Autodesk Inventor part; units mm, degrees
ref_plane "YZ Plane" through (0, 0, 0) normal (1, 0, 0) x (0, 1, 0)
ref_plane "XZ Plane" through (0, 0, 0) normal (0, 1, 0) x (-1, 0, 0)
ref_plane "XY Plane" through (0, 0, 0) normal (0, 0, 1) x (1, 0, 0)
sketch "スケッチ1" plane through (0, 0, 0) normal (0, 1, 0) x (-1, 0, 0)
  circle A0 centre (0, 0) radius 125
  dimension "d0" = 250
extrude "押し出し1" add sketch "スケッチ1" along normal blind 375
sketch "スケッチ2" plane through (0, 0, 0) normal (0, -1, 0) x (1, 0, 0)
  circle A0 centre (0, 0) radius 125
extrude "押し出し2" cut sketch "スケッチ2" against normal blind 40
sketch "スケッチ3" plane through (0, 40, 0) normal (0, -1, 0) x (1, 0, 0)
  circle A0 centre (0, 0) radius 125
  point P0 (0, 100)
  point P1 (-86.6025, -50)
  point P2 (86.6025, -50)
  dimension "d5" = 100
  dimension "d8" = 360
hole "穴1" at (0, 40, 100) at (-86.6025, 40, -50) at (86.6025, 40, -50) direction (0, 1, 0) diameter 3.2 depth 8
sketch "スケッチ4" plane through (0, 40, 0) normal (0, -1, 0) x (1, 0, 0)
  circle A0 centre (0, 100) radius 1.6
  point P0 (0, 0)
  point P1 (0, 110)
  point P2 (-95.2628, -55)
  point P3 (95.2628, -55)
  dimension "d17" = 10
  dimension "d20" = 360
hole "穴2" at (0, 40, 110) at (-95.2628, 40, -55) at (95.2628, 40, -55) direction (0, 1, 0) diameter 3.2 depth 8
sketch "スケッチ5" plane through (0, 375, 0) normal (0, 1, 0) x (1, 0, 0)
  circle A0 centre (0, 0) radius 120
  dimension "d29" = 240
extrude "押し出し3" cut sketch "スケッチ5" against normal blind 330
sketch "スケッチ6" plane through (0, 45, 0) normal (0, 1, 0) x (1, 0, 0)
  circle A0 centre (0, 0) radius 120
  line L0 (0, -118) -> (-21.8174, -118)
  line L1 (0, -118) -> (21.8174, -118)
  arc A1 (21.8174, -118) -> (-21.8174, -118) centre (0, 0) ccw
  arc A2 (-21.8174, -118) -> (21.8174, -118) centre (0, 0) ccw
  arc A3 (113.0997, 40.1056) -> (91.2823, 77.8944) centre (0, 0) ccw
  line L2 (102.191, 59) -> (91.2823, 77.8944)
  line L3 (102.191, 59) -> (113.0997, 40.1056)
  arc A4 (-91.2823, 77.8944) -> (-113.0997, 40.1056) centre (0, 0) ccw
  line L4 (-102.191, 59) -> (-113.0997, 40.1056)
  line L5 (-102.191, 59) -> (-91.2823, 77.8944)
  point P0 (-91.2823, 77.8944)
  point P1 (-113.0997, 40.1056)
  point P2 (113.0997, 40.1056)
  point P3 (91.2823, 77.8944)
  dimension "d32" = 118
  dimension "d35" = 360
extrude "押し出し4" add sketch "スケッチ6" along normal blind 330 contours L3 L2 A0 | A0 L0 L1 | L5 L4 A0
sketch "スケッチ8" plane through (21.8174, 45, 118) normal (0, 0, -1) x (-1, 0, 0)
  line L0 (43.6348, 0) -> (0, 0)
  point P0 (21.8174, -45)
  point P1 (11.8174, 60)
  point P2 (31.8174, 60)
  point P3 (11.8174, 90)
  point P4 (31.8174, 90)
  dimension "d52" = 30
  dimension "d90" = 60
  dimension "d91" = 60
  dimension "d92" = 30
hole "穴4" at (10, 105, 118) at (-10, 105, 118) at (10, 135, 118) at (-10, 135, 118) direction (0, 0, 1) diameter 3.2 depth 8
sketch "スケッチ11" plane through (113.0997, 45, -40.1056) normal (-0.8660254, 0, 0.5) x (0.5, 0, 0.8660254)
  line L0 (0, 0) -> (-43.6348, 0)
  point P0 (-21.8174, -45)
  point P1 (-31.8174, 60)
  point P2 (-31.8174, 90)
  point P3 (-11.8174, 60)
  point P4 (-11.8174, 90)
  dimension "d65" = 30
  dimension "d95" = 60
  dimension "d96" = 60
  dimension "d98" = 30
hole "穴5" at (97.191, 105, -67.6603) at (97.191, 135, -67.6603) at (107.191, 135, -50.3397) at (107.191, 105, -50.3397) direction (0.8660254, 0, -0.5) diameter 3.2 depth 8
sketch "スケッチ12" plane through (0, 375, 0) normal (0, 1, 0) x (1, 0, 0)
  circle A0 centre (0, 0) radius 121.5
  dimension "d73" = 243
extrude "押し出し6" cut sketch "スケッチ12" against normal blind 330
sketch "スケッチ13" plane through (0, 375, 0) normal (0, 1, 0) x (1, 0, 0)
  circle A0 centre (0, 0) radius 125
  line L0 (0, -125) -> (0, 0)
  line L1 (0, 0) -> (108.2532, 62.5)
  arc A1 (0, -125) -> (108.2532, 62.5) centre (0, 0) ccw
  circle A2 centre (0, 0) radius 125
  dimension "d76" = 125
  dimension "d77" = 120
extrude "押し出し7" cut sketch "スケッチ13" against normal blind 400 contours L1 L0 A0 picked at (69.3351, 45.9431)
sketch "スケッチ14" plane through (0, 45, 0) normal (0, 1, 0) x (1, 0, 0)
  line L0 (0, 0) -> (85.2169, 49.2)
  line L1 (0, -111.6) -> (0, -121.5)
  circle A0 centre (0, 0) radius 121.5
extrude "押し出し8" cut sketch "スケッチ14" against normal blind 400
sketch "スケッチ15" plane through (0, 40, 0) normal (0, -1, 0) x (1, 0, 0)
  line L0 (0, 0) -> (105.2221, 60.75)
  arc A0 (105.2221, -60.75) -> (0, 121.5) centre (0, 0) ccw
  line L1 (0, 0) -> (121.5, 0) construction
  line L2 (102.9357, 59.43) -> (115.531, 37.6143)
  line L3 (102.9357, 59.43) -> (90.3404, 81.2456)
  dimension "d82" = 30
extrude "押し出し9" add sketch "スケッチ15" against normal blind 335
sketch "スケッチ17" plane through (0, 40, 0) normal (0, -1, 0) x (1, 0, 0)
  circle A0 centre (0, 0) radius 125
extrude "押し出し11" cut sketch "スケッチ17" against normal blind 5
sketch "スケッチ19" plane through (0, 375, 0) normal (0, 1, 0) x (1, 0, 0)
  arc A0 (115.531, -37.6143) -> (105.2221, 60.75) centre (0, 0) ccw
  line L0 (115.531, -37.6143) -> (90.3404, -81.2456)
  line L1 (115.531, -37.6143) -> (90.3404, -81.2456)
  line L2 (90.3404, -81.2456) -> (81.6802, -76.2456)
  line L3 (115.531, -37.6143) -> (106.8708, -32.6143)
  line L4 (106.8708, -32.6143) -> (81.6802, -76.2456)
  dimension "d104" = 10
extrude "押し出し13" add sketch "スケッチ19" against normal blind 330
sketch "スケッチ21" plane through (0, 375, 0) normal (0, 1, 0) x (1, 0, 0)
  circle A0 centre (0, 0) radius 125
extrude "押し出し15" cut sketch "スケッチ21" against normal blind 230
fillet "フィレット1" radius 8 2 edges at (115.531, 95, 37.6143) (90.3404, 95, 81.2456)
sketch "スケッチ22" plane through (106.8708, 45, 32.6143) normal (-0.8660254, 0, -0.5) x (-0.5, 0, 0.8660254)
  line L0 (50.3812, 100) -> (0, 100)
  line L1 (25.1906, 85) -> (25.1906, 80.9836)
  point P0 (25.1906, -45)
  point P1 (10.1906, 85)
  point P2 (10.1906, 70)
  point P3 (40.1906, 85)
  point P4 (40.1906, 70)
  dimension "d112" = 15
  dimension "d113" = 15
  dimension "d114" = 15
hole "穴6" at (94.2755, 130, 54.43) at (101.7755, 130, 41.4396) at (101.7755, 115, 41.4396) at (86.7755, 130, 67.4204) at (86.7755, 115, 67.4204) direction (0.8660254, 0, 0.5) diameter 2.6 depth 10
sketch "スケッチ23" plane through (0, 45, 0) normal (0, -1, 0) x (1, 0, 0)
  line L0 (81.6802, 76.2456) -> (106.8708, 32.6143)
  arc A0 (118.386, 27.3315) -> (106.8708, 32.6143) centre (110.591, 25.5319) ccw
  line L1 (106.8708, 32.6143) -> (94.2755, 54.4299)
  line L2 (102.2857, 60.5558) -> (93.6255, 55.5558)
  line L3 (94.2755, 54.43) -> (101.2037, 58.43)
  line L4 (103.5857, 58.3041) -> (94.9255, 53.3041)
  line L5 (94.2755, 54.43) -> (102.2755, 54.43) construction
  point P0 (0, 0)
  dimension "d124" = 25.1905
  dimension "d126" = 8
  dimension "d127" = 30
hole "穴7" at (101.2037, 45, 58.43) direction (0, 1, 0) diameter 2.6 depth 10
sketch "スケッチ24" plane through (0, 45, 0) normal (0, -1, 0) x (1, 0, 0)
  circle A0 centre (101.2037, 58.43) radius 1.3
  line L0 (101.2037, 58.43) -> (96.2037, 67.0902)
  line L1 (94.7857, 73.5462) -> (86.1255, 68.5462)
  line L2 (101.2037, 58.43) -> (111.2037, 58.43) construction
  line L3 (96.2037, 67.0902) -> (106.2037, 49.7697)
  point P0 (0, 0)
  dimension "d135" = 10
  dimension "d136" = 120
  dimension "d137" = 20
hole "穴8" at (96.2037, 45, 67.0902) at (106.2037, 45, 49.7697) direction (0, 1, 0) diameter 2.6 depth 10
sketch "スケッチ27" plane through (0, 145, 0) normal (0, 1, 0) x (1, 0, 0)
  circle A0 centre (101.2037, -58.43) radius 1.3
  circle A1 centre (96.2037, -67.0902) radius 1.3
  circle A2 centre (106.2037, -49.7697) radius 1.3
  point P0 (0, 0)
hole "穴10" at (101.2037, 145, 58.43) at (96.2037, 145, 67.0902) at (106.2037, 145, 49.7697) direction (0, -1, 0) diameter 2.7 depth 10
properties part number "newbody5" material "PC/ABS プラスチック"
Geometry check sheet. Reference: the model listing, model coordinates, mm. A direction names the side the tool comes from. Give positions to 0.01 mm unless a question says otherwise; leave off trailing zeros. Loops run counter-clockwise (first coordinate to the right, second up) from the corner with the lowest first, then second, coordinate; pieces in that order, holes last. Notation, with made-up numbers: (66, 89) -> (99, 89) arc R25 ccw to (99, 124) -> close; hole circle Ø5 at (-15, 8). An arc over 180 degrees is marked (long way). Answer in a Markdown table with one row per item. Add a question column.
1) Cross-section at C-C on x = 48. Record the boundary of the cut face in (y, z), and give its area (3 significant figures).
2) Gauge pin test, flat ends, axial feed: P1, Ø2, axis at x = 101, z = 58.5, coming from the +Y side; P2, Ø1.5, axis at x = 82.5, y = 58, coming from the -Z side; P3, Ø12, axis at y = 70, z = 41, coming from the +X side. Record the tip position at first contact, or that the pin passes through.
3) Cross-section at A-A on y = 63. Record the boundary of the cut face in (x, z).
4) Material ranges on probe 1 along Y at (x, z) = (94, 72); probe 2 along Y at (x, z) = (10, 122); probe 3 along X at (y, z) = (98, -2.5) (3 decimals), recorded low to high. Write a range as from..to.
5) Draft check along Y on faces 1 (the face through (99, 45, 52)), 2 (the face through (85.357, 94.3, 82.166)), 3 (the face through (110.723, 104.14, -53.937)), 4 (the face through (99, 145, 52)). Enter one of: pulls with the +Y half, pulls with the -Y half, needs draft (parallel to the pull), parting line crosses it, or undercut.
6) Set-up check for faces 5 (the face through (98.47, 131.24, 57.3)), 6 (the face through (114.022, 94.3, 32.753)): record each of +Z, -Z, +X, -X, +Y, -Y from which the full face is reachable in a straight line by a thin tool's end or side.
7) Cross-section at B-B on z = 92. Record the boundary of the cut face in (x, y).
Outcome:
| question | item | result |
|---|---|---|
| 1 | outline | (45, 111.62) -> (145, 111.62) -> (145, 115.42) -> (45, 115.42) -> close |
| 1 | area | 380 mm^2 |
| 2 | P1 | stops at y = 135 |
| 2 | P2 | stops at z = 73.53 |
| 2 | P3 | stops at x = 120 |
| 3 | outline | (0, 121.5) arc R121.5 cw to (82.86, 88.86) arc R8 cw to (81.68, 76.25) -> (106.87, 32.61) arc R8 cw to (118.39, 27.32) arc R121.5 cw to (105.22, -60.75) -> (108.25, -62.5) arc R125 ccw to (0, 125) -> close |
| 4 | probe 1 | y = 45..113.75, 116.25..128.75, 131.25..145 |
| 4 | probe 2 | y = 45..103.4, 106.6..133.4, 136.6..145 |
| 4 | probe 3 | x = 121.474..124.975 |
| 5 | face 1 | pulls with the -Y half |
| 5 | face 2 | needs draft |
| 5 | face 3 | undercut |
| 5 | face 4 | pulls with the +Y half |
| 6 | face 5 | none |
| 6 | face 6 | +Y, -Y |
| 7 | outline | (79.36, 45) -> (84.62, 45) -> (84.62, 145) -> (79.36, 145) -> close |
